Geometry: final body of the model. Coordinates: model frame, mm. A direction names the side the tool comes from. Give positions to 0.01 mm unless a question says otherwise; leave off trailing zeros. One line per question, with ' | ' between items.
from build123d import *

# Parameters (mm, degrees)
SKETCH1_W           = 2209.8
SKETCH1_H           = 284.1625
BOSS_EXTRUDE1_DEPTH = 50.8
SKETCH2_R           = 9.525
CUT_EXTRUDE1_DEPTH  = 1119.621317337
SKETCH3_W           = 85.725
SKETCH3_H           = 44.45
CUT_EXTRUDE2_DEPTH  = 25.4


with BuildPart() as part:
    # Sketch1 → Boss-Extrude1 (new, symmetric)
    with BuildSketch(Plane(origin=(0, 0, 0), x_dir=(1, 0, 0), z_dir=(0, 1, 0))):
        Rectangle(SKETCH1_W, SKETCH1_H)
    extrude(amount=BOSS_EXTRUDE1_DEPTH, both=True)

    # Sketch2 → Cut-Extrude1 (cut, through all)
    with BuildSketch(Plane(origin=(0, 50.8, 0), x_dir=(1, 0, 0), z_dir=(0, 1, 0))):
        with Locations(Location((-946.15, -62.70625, 0), (0, 0, 270))):
            Circle(SKETCH2_R)
        with Locations(Location((-520.7, 42.06875, 0), (0, 0, 270))):
            Circle(SKETCH2_R)
        with Locations(Location((-139.7, 42.06875, 0), (0, 0, 270))):
            Circle(SKETCH2_R)
        with Locations(Location((241.3, 42.06875, 0), (0, 0, 270))):
            Circle(SKETCH2_R)
        with Locations(Location((622.3, 42.06875, 0), (0, 0, 270))):
            Circle(SKETCH2_R)
    extrude(amount=-CUT_EXTRUDE1_DEPTH, mode=Mode.SUBTRACT)

    # Sketch3 → Cut-Extrude2 (cut)
    with BuildSketch(Plane.XZ.offset(50.8)):
        with Locations((531.8125, -91.28125)):
            Rectangle(SKETCH3_W, SKETCH3_H)
        with Locations((-661.9875, -91.28125)):
            Rectangle(SKETCH3_W, SKETCH3_H)
    extrude(amount=-CUT_EXTRUDE2_DEPTH, mode=Mode.SUBTRACT)


solid = part.part
1) Set-up query: faces 4 (the flat face through (1104.9, 1, 2)), 5 (the flat face through (531, -25.4, -91)). Return all of +Z, -Z, +X, -X, +Y, -Y with unobstructed straight access to the full face (end or side cutting, diameter ignored); none if empty.
Check result:
face 4: +Z, -Z, +X, +Y, -Y | face 5: -Y
2) Material intervals for probe 1 along Z at (x, y) = (622.3, -29.5); probe 2 along X at (y, z) = (45.5, 66.5), sorted ascending. Write a range as from..to.
Check result:
probe 1: z = -142.08..-51.59, -32.54..142.08 | probe 2: x = -1104.9..-954.89, -937.41..1104.9
3) Pull-direction query (Z, two-part tool) for faces 1 (the flat face through (-15, 1, 142.081)), 2 (the flat face through (-663, -25.4, -91)), 3 (the flat face through (-15, -50.8, -2)); classes: +Z half, -Z half, draft (parallel to the pull), parting line (faces both ways), or undercut.
Check result:
face 1: +Z half | face 2: undercut | face 3: draft
